For this review, take the finished solid that the model builds, in its own axes (mm). Round coordinates to 2 decimals unless told otherwise and drop trailing zeros. Loops run counter-clockwise (first coordinate to the right, second up) from the corner with the lowest first, then second, coordinate; pieces in that order, holes last.
1. Consider section C-C on x = 73. State the section outline as (y, z) points.
2. To check wall thickness, follow line 1 along X through (y, z) = (0, 6.25); line 2 along X through (y, z) = (0.25, 1.75); line 3 along X through (y, z) = (0, 2.5). State the ranges of each line that lie inside material, in increasing order.
3. Consider section A-A on x = 39.5. State the section outline as (y, z) points, then the cut area to 3 significant figures.
4. Clearance check with flat-ended pins moving along their axes: pin 1 Ø5 at (x, z) = (23, 5.5) entering from -Y; pin 2 Ø2 at (x, z) = (51.5, -3.5) entering from -Y; pin 3 Ø1.5 at (x, y) = (12, -3) entering from +Z. State where each tip first meets the part, or that it passes through.
5. Consider section B-B on z = 3.75. State how many separate pieces and enclosed holes the cut face has, then the cut area to 3 significant figures.
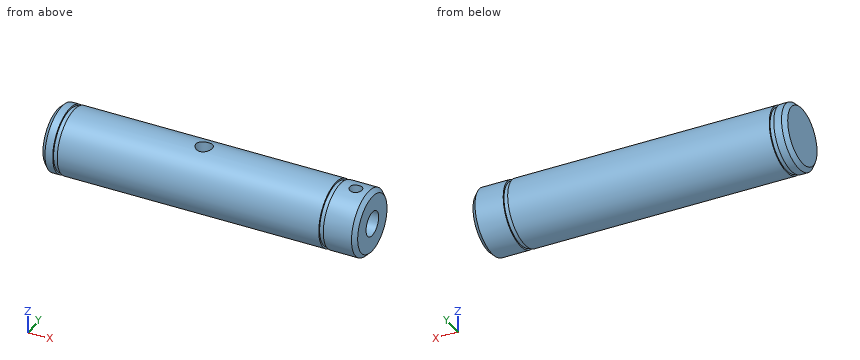
Autodesk Inventor part; units mm, degrees
ref_plane "YZ Plane" through (0, 0, 0) normal (1, 0, 0) x (0, 1, 0)
ref_plane "XZ Plane" through (0, 0, 0) normal (0, 1, 0) x (-1, 0, 0)
ref_plane "XY Plane" through (0, 0, 0) normal (0, 0, 1) x (1, 0, 0)
sketch "Sketch1" plane through (0, 0, 0) normal (0, 0, 1) x (1, 0, 0)
  line L0 (0, 0) -> (77, 0)
  line L1 (77, 0) -> (77, 8)
  line L2 (77, 8) -> (0, 8)
  line L3 (0, 8) -> (0, 0)
  line L4 (68, 8) -> (69.1, 8)
  line L5 (69.1, 8) -> (69.1, 7.6)
  line L6 (69.1, 7.6) -> (68, 7.6)
  line L7 (68, 7.6) -> (68, 8)
  line L8 (38.5, 8) -> (38.5, 0)
  line L9 (77, 0) -> (57, 0)
  line L10 (57, 0) -> (57, 3)
  line L11 (57, 3) -> (77, 3)
  line L12 (77, 3) -> (77, 0)
  line L13 (2.9, 8) -> (4, 8)
  line L14 (4, 8) -> (4, 7.6)
  line L15 (4, 7.6) -> (2.9, 7.6)
  line L16 (2.9, 7.6) -> (2.9, 8)
  point P0 (68.55, 7.6)
  point P1 (69.1, 7.8)
  point P2 (57, 0)
  point P3 (77, 3)
  point P4 (69.1, 8)
  point P5 (4, 8)
  dimension "d0" = 77
  dimension "d1" = 8
  dimension "d2" = 1.1
  dimension "d3" = 7.6
  dimension "d4" = 7.9
  dimension "d5" = 20
  dimension "d6" = 3
  dimension "d8" = 1.1
  dimension "d9" = 7.6
  dimension "d10" = 2.9
revolve "Revolution1" add sketch "Sketch1" angle 360 about axis through (0, 0, 0) along (1, 0, 0) contours L3 L2 L16 L15 L14 L8 L0 | L8 L2 L7 L6 L5 L1 L11 L10 L0
sketch "Sketch2" plane through (0, 0, 0) normal (0, 0, 1) x (1, 0, 0)
  line L0 (77, -3) -> (77, 3)
  line L1 (57, -3) -> (57, 3)
  circle A0 centre (73, 0) radius 1.5
  circle A1 centre (35.8607, 0) radius 2
  point P0 (0, 0)
  dimension "d11" = 3
  dimension "d12" = 4
  dimension "d18" = 4
extrude "Extrusion1" cut sketch "Sketch2" along normal blind 10
chamfer "Chamfer1" distance 1 angle 45 2 edges at (0, -8, 0) (77, -8, 0)
thread "Thread1"
thread "Thread2"
properties part number "shaft potmeter" material "Stainless Steel"
Resolved:
1. outline: (-1.5, 2.6) - (-1.5, 7.86) arc R8 ccw (long way) to (1.5, 7.86) - (1.5, 2.6) arc R3 cw (long way) to start
2. line 1: x = 0 to 33.86, 37.86 to 71.5, 74.5 to 77
2. line 2: x = 0 to 33.88, 37.85 to 57
2. line 3: x = 0 to 33.86, 37.86 to 57
3. outline: circle Ø16 at (0, 0)
3. area: 201 mm2
4. pin 1: stops at y = -7.42
4. pin 2: stops at y = -7.6
4. pin 3: stops at z = 7.68
5. separate pieces: 1
5. enclosed holes: 2
5. area: 1,060 mm2
